Here's how the part is built. I have some questions about the finished solid (model axes, mm). Face numbers are marked on the shaded views. Coordinates: 2 decimals unless noted, no trailing zeros. Write each loop counter-clockwise with the first axis right and the second up, starting at its lowest first coordinate (ties: lowest second). Pieces come first, ordered by that corner, then holes.
(1) Imagine slicing it at B-B, the plane y = 0. List the corners of the cut face in (x, z) for me.
(2) For pin 1 Ø6 at (x, z) = (-10.5, 36) entering from +Y; pin 2 Ø2 at (x, z) = (15.5, 110) entering from +Y; pin 3 Ø1 at (y, z) = (51, 108) entering from -X, each with a flat end and sliding along its axis, tell me the tip position at first contact or that it passes through.
(3) Please list where these lines run through material, in increasing order: probe 1 along Y at (x, z) = (0, 56); probe 2 along Z at (x, y) = (-36, 43); probe 3 along Y at (x, z) = (-11.5, 25).
(4) Imagine slicing it at A-A, the plane z = 126.5. List the corners of the cut face in (x, y) for me.
(5) Thinking about a two-plate mould opening in Y: for the marked faces 1, 2 and 3, which applies, released by +Y, released by -Y, zero draft, split by the parting line, or undercut?
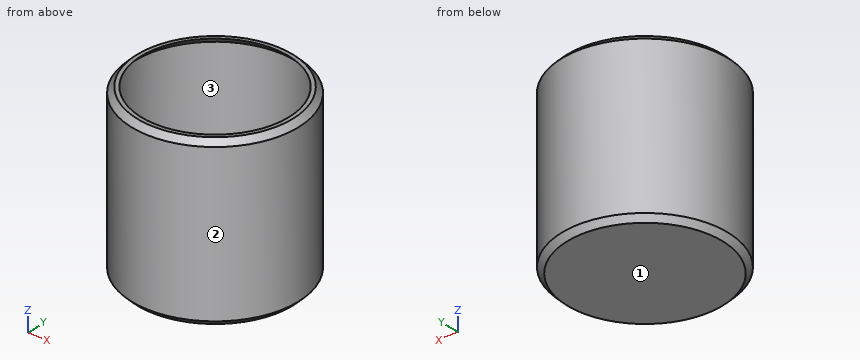
```python
from build123d import *

# Parameters (mm, degrees)
F0_R     = 76.2
F1_DEPTH = 152.4
F2_SIZE  = 5.08
F3_T     = -2.54


with BuildPart() as f1:
    # F0 (on Top) → F1 (new body)
    with BuildSketch(Plane.XY):
        Circle(F0_R)
    extrude(amount=F1_DEPTH)

    # F2
    f2_edges = [f1.edges().sort_by_distance(p)[0] for p in [
        (-76.2, 0, 152.4),
        (76.2, 0, 76.2),
        (-76.2, 0, 0),
    ]]
    chamfer(f2_edges, length=F2_SIZE)

    # F3
    f3_openings = [f1.faces().sort_by_distance(p)[0] for p in [
        (0, 0, 152.4),
    ]]
    offset(amount=F3_T, openings=f3_openings)


solid = f1.part
```
Recorded:
1. outline: (-76.2, 5.08) - (-71.12, 0) - (71.12, 0) - (76.2, 5.08) - (76.2, 147.32) - (71.12, 152.4) - (67.53, 152.4) - (73.66, 146.27) - (73.66, 6.13) - (70.07, 2.54) - (-70.07, 2.54) - (-73.66, 6.13) - (-73.66, 146.27) - (-67.53, 152.4) - (-71.12, 152.4) - (-76.2, 147.32) - close
2. pin 1: stops at y = 75.83
2. pin 2: stops at y = 74.81
2. pin 3: stops at x = -57.06
3. probe 1: y = -76.2 to -73.66, 73.66 to 76.2
3. probe 2: z = 0 to 2.54
3. probe 3: y = -75.33 to -72.76, 72.76 to 75.33
4. outline: circle Ø152.4 at (0, 0); hole circle Ø147.32 at (0, 0)
5. face 1: zero draft
5. face 2: split by the parting line
5. face 3: undercut
